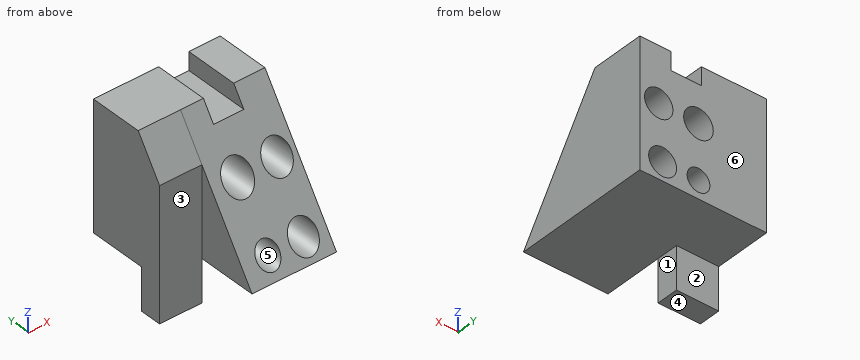
```python
from build123d import *

# Parameters (mm, degrees)
F1_DEPTH = 50.8
F2_W     = 18.229121
F2_H     = 10.856584
F3_DEPTH = 63.5
F4_R     = 8.548371
F4_R_2   = 8.901735
F4_R_3   = 6.849237
F4_R_4   = 8.384756
F5_DEPTH = 109.474
F7_DEPTH = 25.4
F9_DEPTH = 25.4


with BuildPart() as f1:
    # F0 (on Right) → F1 (new body)
    with BuildSketch(Plane.YZ):
        Polygon((-46.180889, -24.980081), (37.1475, -24.980081), (37.1475, 51.52718), (5.069758, 51.52718), align=None)
    extrude(amount=F1_DEPTH)

    # F2 (on face) → F3 (cut)
    with BuildSketch(Plane(origin=(0, 37.1475, 0), x_dir=(-1, 0, 0), z_dir=(0, 1, 0))):
        with Locations((-22.876179, 46.098888)):
            Rectangle(F2_W, F2_H)
    extrude(amount=-F3_DEPTH, mode=Mode.SUBTRACT)

    # F4 (on face) → F5 (cut)
    with BuildSketch(Plane(origin=(0, 37.1475, 0), x_dir=(-1, 0, 0), z_dir=(0, 1, 0))):
        with Locations((-39.41891, 18.436231)):
            Circle(F4_R)
        with Locations((-15.524367, 18.102858)):
            Circle(F4_R_2)
        with Locations((-15.524367, -14.255895)):
            Circle(F4_R_3)
        with Locations((-37.082806, -13.922811)):
            Circle(F4_R_4)
    extrude(amount=-F5_DEPTH, mode=Mode.SUBTRACT)

    # F6 (on face) → F7 (join)
    with BuildSketch(Plane(origin=(0, 0, 0), x_dir=(0, -1, 0), z_dir=(-1, 0, 0))):
        Polygon((-5.069758, 51.52718), (-37.1475, 51.52718), (-37.1475, -24.980081), (10.234666, -24.980081), (10.234666, 28.680648), align=None)
    extrude(amount=F7_DEPTH)

    # F8 (on face) → F9 (join)
    with BuildSketch(Plane(origin=(0, 0, -24.980081), x_dir=(1, 0, 0), z_dir=(0, 0, -1))):
        Polygon((-25.4, 10.234666), (-25.4, -2.907777), (0, -2.907777), (0, 10.234666), (-21.744397, 10.234666), align=None)
    extrude(amount=F9_DEPTH)


solid = f1.part
```
The listing builds one solid part. Answer for the finished solid, in the listing's coordinates (mm). Face numbers are marked on the shaded views. A direction names the side the tool comes from. Round coordinates to 2 decimals unless told otherwise and drop trailing zeros. Order: outer loops, then holes, each group sorted by start corner. A loop starts at its lowest first (then second) coordinate and runs counter-clockwise, first axis right, second up. Notation, with made-up numbers: (0.25, 51.5) -> (13.25, 51.5) arc R21 ccw to (13.25, 70.5) -> close; hole circle Ø11 at (3.5, -18.75). An arc over 180 degrees is marked (long way). Answer as CSV lines item,"result". Start each with the question number.
(1) Find the intervals of material crossed by probe 1 along X at (y, z) = (-18.5, -14); probe 2 along X at (y, z) = (33, -15.5); probe 3 along Z at (x, y) = (38, 26), in increasing order. Write a range as from..to.
(2) The part is cut by section A-A (z = 24). Determine the outline of the cut face in (x, y), then the cut area to 3 significant figures.
(3) The part is cut by section D-D (x = -19.5). Determine the outline of the cut face in (y, z).
(4) A tool of negligible diameter and unlimited length cuts with its end or side. For the marked faces 1, 2 and 3, from which of +Z, -Z, +X, -X, +Y, -Y can it reach the whole face along a straight path? Write none if from no direction.
(5) For a pull along Z with two mould halves and no side action, classify the marked faces 4, 5 and 6 as +Z half, -Z half, draft (parallel to the pull), parting line (faces both ways), or undercut.
(6) Flat-ended cylindrical pins translate along their axes: pin 1 Ø12 at (x, y) = (27, -17) entering from +Z; pin 2 Ø20.5 at (x, z) = (15.52, 18.1) entering from -Y; pin 3 Ø23 at (x, y) = (24.5, 16) entering from -Z. Find the tip coordinate at first contact, or state that the pin passes through.
(7) The part is cut by section C-C (y = -8.5). Determine the outline of the cut face in (x, z), then the cut area to 3 significant figures.
(8) The part is cut by section B-B (x = 10.5). Determine the outline of the cut face in (y, z).
Evaluation:
1,probe 1,"0..8.68, 22.37..28.7, 45.47..50.8"
1,probe 2,"-25.4..8.79, 22.26..28.85, 45.32..50.8"
1,probe 3,"-24.98..-22.26, -5.59..10.01, 26.87..51.53"
2,outline,"(-25.4, -10.23) -> (0, -10.23) -> (0, -13.37) -> (8.86, -13.37) -> (8.86, 37.15) -> (-25.4, 37.15) -> close; (22.19, -13.37) -> (32.93, -13.37) -> (32.93, 37.15) -> (22.19, 37.15) -> close; (45.91, -13.37) -> (50.8, -13.37) -> (50.8, 37.15) -> (45.91, 37.15) -> close"
2,area,"2,440 mm²"
3,outline,"(-10.23, -50.38) -> (2.91, -50.38) -> (2.91, -24.98) -> (37.15, -24.98) -> (37.15, 51.53) -> (5.07, 51.53) -> (-10.23, 28.68) -> close"
4,face 1,"-Z, +X, +Y, -Y"
4,face 2,"-Z, +X, -X, +Y"
4,face 3,"+Z, -Z, -X, -Y"
5,face 4,"-Z half"
5,face 5,"undercut"
5,face 6,"draft"
6,pin 1,"z = 27.54"
6,pin 2,"y = -24.19"
6,pin 3,"z = -24.98"
7,outline,"(-25.4, -50.38) -> (0, -50.38) -> (0, -24.98) -> (50.8, -24.98) -> (50.8, 31.27) -> (-25.4, 31.27) -> close; hole circle Ø17.8 at (15.52, 18.1); hole circle Ø13.7 at (15.52, -14.26); hole circle Ø16.77 at (37.08, -13.92); hole circle Ø17.1 at (39.42, 18.44)"
7,area,"4,080 mm²"
8,outline,"(-46.18, -24.98) -> (37.15, -24.98) -> (37.15, -18.91) -> (-42.12, -18.91) -> close; (-35.88, -9.6) -> (37.15, -9.6) -> (37.15, 10.75) -> (-22.24, 10.75) -> close; (-12.4, 25.45) -> (37.15, 25.45) -> (37.15, 51.53) -> (5.07, 51.53) -> close"
